```python
from build123d import *

# Parameters (mm, degrees)
BOSS_EXTRUDE1_DEPTH = 10
SKETCH1_4_W         = 16.4
SKETCH1_4_H         = 37.6
BOSS_EXTRUDE2_DEPTH = 4
SKETCH3_W           = 18
SKETCH3_H           = 5
CUT_EXTRUDE2_DEPTH  = 70.74955197
FILLET2_R           = 1
FILLET3_R           = 2


with BuildPart() as part:
    # Sketch1 → Boss-Extrude1 (new body)
    with BuildSketch(Plane(origin=(0, 0, 0), x_dir=(1, 0, 0), z_dir=(0, 1, 0))):
        with BuildLine():
            Line((-9, -21.5), (9, -21.5))
            ThreePointArc((9, -21.5), (10.414213562, -20.914213562), (11, -19.5))
            Line((11, -19.5), (11, 19.5))
            ThreePointArc((11, 19.5), (10.414213562, 20.914213562), (9, 21.5))
            Line((9, 21.5), (-9, 21.5))
            ThreePointArc((-9, 21.5), (-10.414213562, 20.914213562), (-11, 19.5))
            Line((-11, 19.5), (-11, -19.5))
            ThreePointArc((-11, -19.5), (-10.414213562, -20.914213562), (-9, -21.5))
        make_face()
    extrude(amount=BOSS_EXTRUDE1_DEPTH)

    # Sketch1<4> → Boss-Extrude2 (add)
    with BuildSketch(Plane(origin=(0, 0, 0), x_dir=(1, 0, 0), z_dir=(0, 1, 0))):
        Rectangle(SKETCH1_4_W, SKETCH1_4_H)
    extrude(amount=-BOSS_EXTRUDE2_DEPTH)

    # Sketch3 → Cut-Extrude2 (cut, through all)
    with BuildSketch(Plane(origin=(-43, 0, -21.5), x_dir=(1, 0, 0), z_dir=(0, 0, 1))):
        with Locations((43, 5)):
            Rectangle(SKETCH3_W, SKETCH3_H)
    extrude(amount=CUT_EXTRUDE2_DEPTH, mode=Mode.SUBTRACT)

    # Fillet2
    fillet2_edges = [part.edges().sort_by_distance(p)[0] for p in [
        (10.414213562, 10, -20.914213562),
        (11, 10, 0),
        (10.414213562, 10, 20.914213562),
        (0, 10, 21.5),
        (-10.414213562, 10, 20.914213562),
        (-11, 10, 0),
        (-10.414213562, 10, -20.914213562),
        (0, 10, -21.5),
    ]]
    fillet(fillet2_edges, radius=FILLET2_R)

    # Fillet3
    # the kernel refuses this fillet: 2 mm, written as the material it takes off along each edge
    with BuildSketch(Plane(origin=(9, 2.5, -21.5), x_dir=(0, -1, 0), z_dir=(-1, 0, 0))) as fillet3_piece_1:
        with BuildLine():
            CenterArc((FILLET3_R, FILLET3_R), FILLET3_R, 180, 90)
            Line((0, FILLET3_R), (0, 0))
            Line((0, 0), (FILLET3_R, 0))
        make_face()
    extrude(amount=18, mode=Mode.SUBTRACT)
    with BuildSketch(Plane(origin=(9, 2.5, 21.5), x_dir=(0, -1, 0), z_dir=(-1, 0, 0))) as fillet3_piece_2:
        with BuildLine():
            CenterArc((FILLET3_R, -FILLET3_R), FILLET3_R, 90, 90)
            Line((0, -FILLET3_R), (0, 0))
            Line((0, 0), (FILLET3_R, 0))
        make_face()
    extrude(amount=18, mode=Mode.SUBTRACT)


solid = part.part
```
Could you check a few things on this model? Use its own coordinates, in mm. A direction names the side the tool comes from. Give positions to 0.01 mm unless a question says otherwise; leave off trailing zeros. Write each loop counter-clockwise with the first axis right and the second up, starting at its lowest first coordinate (ties: lowest second). Pieces come first, ordered by that corner, then holes. Notation, with made-up numbers: (47.25, 5.5) - (54.25, 5.5) arc R4 cw to (54.25, 12.5) - close; hole circle Ø3 at (74, 33.25). An arc over 180 degrees is marked (long way). One line per item, written item: value. Start each with the question number.
Item 1: Please list where these lines run through material, in increasing order: line 1 (Y direction, x = 6.75, z = 3.5); line 2 (Y direction, x = -8.5, z = 17); line 3 (X direction, y = 7, z = -4). Write a range as from..to.
Item 2: I'm going to push flat-ended pins straight in: pin 1 (3 mm diameter, centred on x = -4, y = -2.5, fed in from -Z); pin 2 (1.2 mm diameter, centred on x = -1.5, y = -2, fed in from +Z); pin 3 (2 mm diameter, centred on y = -2, z = -0.5, fed in from -X). Where does each tip first touch, or does it pass through?
Item 3: Imagine slicing it at A-A, the plane x = -1.25. List the corners of the cut face in (y, z) for me.
Item 4: Imagine slicing it at C-C, the plane y = 6. List the corners of the cut face in (x, z) for me.
Item 5: Imagine slicing it at D-D, the plane y = 2. List the corners of the cut face in (x, z) for me, and give its area (3 significant figures).
Item 6: Which directions (+Z, -Z, +X, -X, +Y, -Y) give clear straight access to the entire face, cutting with the end or side of a thin tool? Please do faces 4 (the face through (0, -2, 18.8)), 5 (the face through (-8.2, -2, 0)), 6 (the face through (8.2, -2, 0)), 7 (the face through (0, 7.5, 0)).
Item 7: Imagine slicing it at B-B, the plane z = 11. List the corners of the cut face in (x, y) for me, and give its area (3 significant figures).
Item 8: If we mould it in two halves opening along X, with no side actions, what happens to faces 1 (the face through (0.13, 1.9, 20.93)), 2 (the face through (11, 4, 0)), 3 (the face through (0, -2, -18.8))? For each: +X half, -X half, draft (parallel to the pull), parting line (faces both ways), or undercut.
Geometry says:
1. line 1: -4..2.5, 7.5..10
1. line 2: 0..2.5, 7.5..10
1. line 3: -11..-9, 9..11
2. pin 1: z = -18.8
2. pin 2: z = 18.8
2. pin 3: x = -8.2
3. outline: (-4, -18.8) - (0, -18.8) - (0, -21.5) - (0.5, -21.5) arc R2 ccw to (2.5, -19.5) - (2.5, 19.5) arc R2 ccw to (0.5, 21.5) - (0, 21.5) - (0, 18.8) - (-4, 18.8) - close; (7.5, -21.5) - (9, -21.5) arc R1 ccw to (10, -20.5) - (10, 20.5) arc R1 ccw to (9, 21.5) - (7.5, 21.5) - close
4. outline: (-11, -19.5) arc R2 ccw to (-9, -21.5) - (-9, 21.5) arc R2 ccw to (-11, 19.5) - close; (9, -21.5) arc R2 ccw to (11, -19.5) - (11, 19.5) arc R2 ccw to (9, 21.5) - close
5. outline: (-11, -19.5) arc R2 ccw to (-9, -21.5) - (-9, -20.82) - (9, -20.82) - (9, -21.5) arc R2 ccw to (11, -19.5) - (11, 19.5) arc R2 ccw to (9, 21.5) - (9, 20.82) - (-9, 20.82) - (-9, 21.5) arc R2 ccw to (-11, 19.5) - close
5. area: 918 mm^2
6. face 4: +Z, +X, -X, -Y
6. face 5: +Z, -Z, -X, -Y
6. face 6: +Z, -Z, +X, -Y
6. face 7: +Z, -Z
7. outline: (-11, 0) - (-8.2, 0) - (-8.2, -4) - (8.2, -4) - (8.2, 0) - (11, 0) - (11, 9) arc R1 ccw to (10, 10) - (-10, 10) arc R1 ccw to (-11, 9) - close; hole (-9, 2.5) - (9, 2.5) - (9, 7.5) - (-9, 7.5) - close
7. area: 195 mm^2
8. face 1: undercut
8. face 2: +X half
8. face 3: draft
